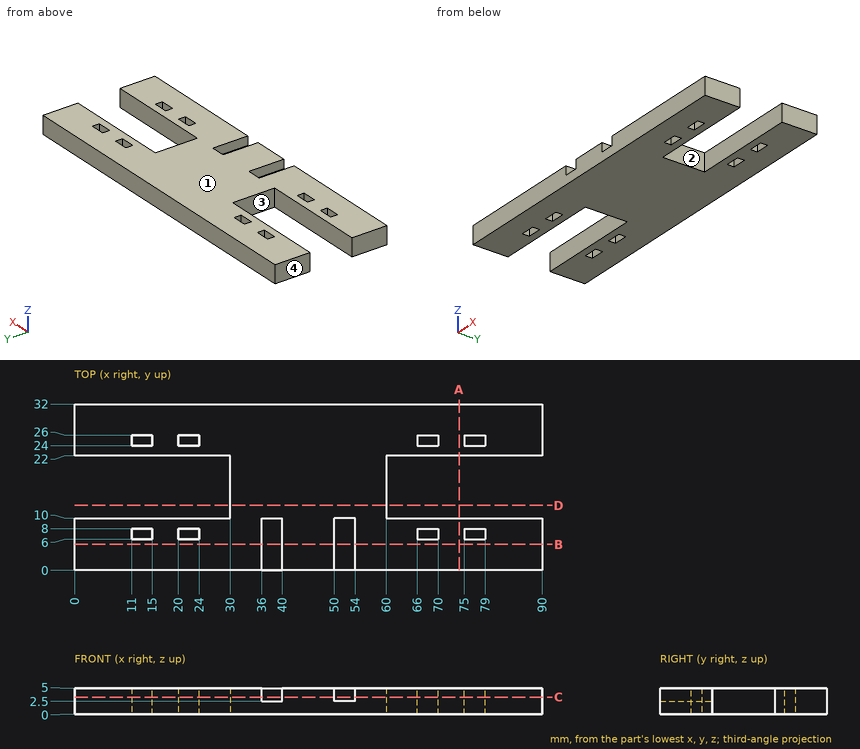
Here's the drawing with two shaded views (mm, measured from the low corner). I have some questions. A direction names the side the tool comes from. Coordinates: 2 decimals unless noted, no trailing zeros. Loops run counter-clockwise (first coordinate to the right, second up) from the corner with the lowest first, then second, coordinate; pieces in that order, holes last. Notation, with made-up numbers: (59.25, 80.5) - (68.25, 80.5) arc R18 ccw to (68.25, 108.5) - close; hole circle Ø11 at (3, -1.75). An arc over 180 degrees is marked (long way). Answer as CSV lines item,"result". Start each with the question number.
1) I need wall thicknesses on line 1 (X direction, y = 1, z = 4.25); line 2 (Y direction, x = 14.5, z = 3.75); line 3 (Y direction, x = 8, z = 2.7). Which ranges of each line are inside material? Lowest first, please. Write a range as from..to.
2) Suppose I cut it at B-B (y = 5). Please give me the cut outline in (x, z).
3) Thinking about a two-plate mould opening in Y: for the marked faces 1 and 2, which applies, pulls with the +Y half, pulls with the -Y half, needs draft (parallel to the pull), parting line crosses it, or undercut?
4) Which directions (+Z, -Z, +X, -X, +Y, -Y) give clear straight access to the entire face, cutting with the end or side of a thin tool? Please do the marked faces 3 and 4.
5) For pin 1 (2 mm diameter, centred on x = 52.5, y = 4, fed in from +Z); pin 2 (2.5 mm diameter, centred on y = 15, z = 3, fed in from +X), each with a flat end and sliding along its axis, tell me the tip position at first contact or that it passes through.
6) Suppose I cut it at D-D (y = 12.5). Please give me the cut outline in (x, z).
7) Suppose I cut it at C-C (z = 3.3). Count the separate pieces of the cut face and the enclosed holes in it, plus the area to 3 significant figures.
8) Suppose I cut it at A-A (x = 74). Please give me the cut outline in (y, z).
Check result:
1,line 1,"x = 0..36, 40..50, 54..90"
1,line 2,"y = 0..6, 8..10, 22..24, 26..32"
1,line 3,"y = 0..10, 22..32"
2,outline,"(0, 0) - (90, 0) - (90, 5) - (54, 5) - (54, 2.5) - (50, 2.5) - (50, 5) - (40, 5) - (40, 2.5) - (36, 2.5) - (36, 5) - (0, 5) - close"
3,face 1,"needs draft"
3,face 2,"undercut"
4,face 3,"+Z, -Z, -X"
4,face 4,"+Z, -Z, -X, +Y, -Y"
5,pin 1,"stops at z = 2.5"
5,pin 2,"stops at x = 60"
6,outline,"(30, 0) - (60, 0) - (60, 5) - (30, 5) - close"
7,separate pieces,"1"
7,enclosed holes,"8"
7,area,"2,020 mm²"
8,outline,"(0, 0) - (10, 0) - (10, 5) - (0, 5) - close; (22, 0) - (32, 0) - (32, 5) - (22, 5) - close"
